The model under review builds one solid part; all positions refer to its coordinate system, in mm. A direction names the side the tool comes from. Give positions to 0.01 mm unless a question says otherwise; leave off trailing zeros. Loops run counter-clockwise (first coordinate to the right, second up) from the corner with the lowest first, then second, coordinate; pieces in that order, holes last. Notation, with made-up numbers: M 16.5,21 L 47.5,21 A19 ccw 47.5,50 Z; hole C -16,-19 d5. An arc over 180 degrees is marked long. One line per item, written item: value. Start each with the question number.
Q1. We need section C-C on y = 0.2. Write out the cut boundary in (x, z), plus the area to 3 significant figures.
Q2. For pin 1 (1.5 mm diameter, centred on y = 0, z = 0, fed in from +X); pin 2 (1.3 mm diameter, centred on x = 6.5, z = 1, fed in from +Y), all flat-tipped, find the tip position at first contact; note any pin that passes through.
Q3. For faces 1 (the face through (-3, -1.15, 0)), 2 (the face through (-0.29, 0.02, -2.23)), 3 (the face through (3, -2, -2.25)), list the 3-axis set-ups (+Z, -Z, +X, -X, +Y, -Y) from which the entire face can be reached by the end or side of a thin tool; tool diameter is ignored.
Q4. We need section A-A on z = 1.8. Write out the cut boundary in (x, y), plus the area to 3 significant figures.
Q5. To check wall thickness, follow line 1 along Y through (x, z) = (4.75, -0.8); line 2 along Z through (x, y) = (-1, -2.6); line 3 along X through (y, z) = (-0.2, 1.1). State the ranges of each line that lie inside material, in increasing order. Write a range as from..to.
Q6. We need section B-B on x = 2.5. Write out the cut boundary in (y, z).
Q7. We need section D-D on z = -1.6. Write out the cut boundary in (x, y), plus the area to 3 significant figures.
```python
from build123d import *

# Parameters (mm, degrees)
SKETCH1_R                = 2.25
BOSS_EXTRUDE1_DEPTH      = 1.15
BOSS_EXTRUDE1_DEPTH_BACK = 1.15
BOSS_EXTRUDE2_DEPTH      = 1.8
CHAMFER2_SIZE            = 1.45
CHAMFER4_SIZE            = 1.45


with BuildPart() as part:
    # Sketch1 → Boss-Extrude1 (new body, two sides)
    with BuildSketch(Plane(origin=(0, 0, 0), x_dir=(1, 0, 0), z_dir=(0, 1, 0))) as boss_extrude1_sk:
        Circle(SKETCH1_R)
    extrude(amount=BOSS_EXTRUDE1_DEPTH)
    extrude(boss_extrude1_sk.sketch, amount=-BOSS_EXTRUDE1_DEPTH_BACK)

    # Sketch2 → Boss-Extrude2 (add)
    with BuildSketch(Plane.XZ.offset(1.15)):
        Polygon((-3.52, 2.25), (3.52, 2.25), (8.82, 2.25), (8.82, -2.25), (3.52, -2.25), (-3.52, -2.25), align=None)
    extrude(amount=BOSS_EXTRUDE2_DEPTH)

    # Chamfer2
    chamfer2_edges = [part.edges().sort_by_distance(p)[0] for p in [
        (2.65, -2.95, 2.25),
    ]]
    chamfer(chamfer2_edges, length=CHAMFER2_SIZE)

    # Chamfer4
    chamfer4_edges = [part.edges().sort_by_distance(p)[0] for p in [
        (-3.52, -2.95, -0.725),
    ]]
    chamfer(chamfer4_edges, length=CHAMFER4_SIZE)


solid = part.part
```
Solved:
1. outline: C 0,0 d4.5
1. area: 15.9 mm2
2. pin 1: x = 2.25
2. pin 2: y = -1.15
3. face 1: -X, +Y
3. face 2: +Y
3. face 3: -Z, +X, -X, +Y, -Y
4. outline: M -3.52,-1.5 L -3.07,-1.95 L 8.82,-1.95 L 8.82,-1.15 L 1.35,-1.15 L 1.35,1.15 L -1.35,1.15 L -1.35,-1.15 L -3.52,-1.15 Z
4. area: 16.0 mm2
5. line 1: -2.95..-1.15
5. line 2: -2.25..1.15
5. line 3: -1.96..1.96
6. outline: M -2.95,-2.25 L -1.15,-2.25 L -1.15,2.25 L -1.5,2.25 L -2.95,0.8 Z
7. outline: M -3.52,-1.5 L -2.07,-2.95 L 8.82,-2.95 L 8.82,-1.15 L 1.58,-1.15 L 1.58,1.15 L -1.58,1.15 L -1.58,-1.15 L -3.52,-1.15 Z
7. area: 28.4 mm2
